Here's how the part is built. I have some questions about the finished solid (model axes, mm). Give positions to 0.01 mm unless a question says otherwise; leave off trailing zeros. Loops run counter-clockwise (first coordinate to the right, second up) from the corner with the lowest first, then second, coordinate; pieces in that order, holes last. Notation, with made-up numbers: (18, -16.75) -> (69, -16.75) arc R12 ccw to (69, 6.25) -> close; hole circle Ø6 at (-11.5, 57). An arc over 180 degrees is marked (long way). Answer in a Markdown table with one row per item. Add a question column.
Item 1: If we section it at D-D (z = 10.5): Write out the boundary of the cut face in (x, y), then the cut area to 3 significant figures.
Item 2: If I drill on line 1 (X direction, y = -1.8, z = 46); line 2 (X direction, y = -0.65, z = 45.5); line 3 (Z direction, x = -18, y = -2.45) (3 decimals), over which ranges is the centre line in solid material (lowest first)?
Item 3: If we section it at C-C (x = 7): Write out the boundary of the cut face in (y, z) (3 decimals).
Item 4: If we section it at B-B (y = -1.2): Write out the boundary of the cut face in (x, z) (3 decimals), then the cut area to 3 significant figures.
Item 5: If we section it at A-A (z = 22.5): Write out the boundary of the cut face in (x, y), then the cut area to 3 significant figures.
Item 6: For P1, Ø1.4, axis at y = -1, z = 11.5, coming from the +X side; P2, Ø1.4, axis at x = -11.5, y = -1, coming from the -Z side; P3, Ø1.4, axis at x = 20, y = -1, coming from the +Z side, each with a flat end and sliding along its axis, tell me the tip position at first contact or that it passes through.
```python
from build123d import *

# Parameters (mm, degrees)
F1_DEPTH = 3.048
F2_SCALE = 0.9


with BuildPart() as f1:
    # F0 (on Front) → F1 (new body)
    with BuildSketch(Plane.XZ):
        Polygon((3.3501721919, 67.3975870013), (0, 67.3975870013), (0, 5.1237931475), (3.3501721919, 5.1237931475), (3.3501721919, 28.9080845579), (24.633621797, 13.3751591098), (27.2410747923, 16.9479306787), (5.6389208675, 32.7134504914), (29.7574140131, 32.7134504914), (29.7574140131, 36.9055655311), (5.6389208675, 36.9055655311), (27.2410747923, 54.3072999545), (24.633621797, 57.5441382825), (3.3501721919, 40.3991378844), align=None)
        Polygon((0, 5.1237931475), (0, 67.3975870013), (-3.3501721919, 67.3975870013), (-3.3501721919, 40.3991378844), (-24.633621797, 57.5441382825), (-27.2410747923, 54.3072999545), (-5.6389208675, 36.9055655311), (-29.7574140131, 36.9055655311), (-29.7574140131, 32.7134504914), (-5.6389208675, 32.7134504914), (-27.2410747923, 16.9479306787), (-24.633621797, 13.3751591098), (-3.3501721919, 28.9080845579), (-3.3501721919, 5.1237931475), align=None)
    extrude(amount=F1_DEPTH)


with BuildPart() as f1_1:
    # F2: moved
    add(f1.part.scale(F2_SCALE))


solid = f1_1.part
```
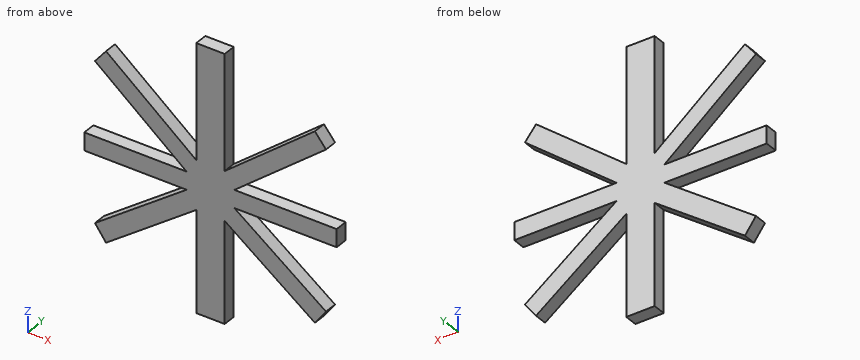
Recorded:
| question | item | result |
|---|---|---|
| 1 | outline | (-3.02, -2.74) -> (3.02, -2.74) -> (3.02, 0) -> (-3.02, 0) -> close |
| 1 | area | 16.5 mm^2 |
| 2 | line 1 | x = -20.95 to -14.98, -3.02 to 3.02, 14.98 to 20.95 |
| 2 | line 2 | x = -20.33 to -14.36, -3.02 to 3.02, 14.36 to 20.33 |
| 2 | line 3 | z = 15.081 to 20.009, 29.442 to 33.215, 43.627 to 48.43 |
| 3 | outline | (-2.743, 23.109) -> (0, 23.109) -> (0, 28.037) -> (-2.743, 28.037) -> close; (-2.743, 29.442) -> (0, 29.442) -> (0, 33.215) -> (-2.743, 33.215) -> close; (-2.743, 34.766) -> (0, 34.766) -> (0, 39.569) -> (-2.743, 39.569) -> close |
| 4 | outline | (-26.782, 29.442) -> (-5.075, 29.442) -> (-24.517, 15.253) -> (-22.17, 12.038) -> (-3.015, 26.017) -> (-3.015, 4.611) -> (3.015, 4.611) -> (3.015, 26.017) -> (22.17, 12.038) -> (24.517, 15.253) -> (5.075, 29.442) -> (26.782, 29.442) -> (26.782, 33.215) -> (5.075, 33.215) -> (24.517, 48.877) -> (22.17, 51.79) -> (3.015, 36.359) -> (3.015, 60.658) -> (-3.015, 60.658) -> (-3.015, 36.359) -> (-22.17, 51.79) -> (-24.517, 48.877) -> (-5.075, 33.215) -> (-26.782, 33.215) -> close |
| 4 | area | 906 mm^2 |
| 5 | outline | (-14.59, -2.74) -> (-7.83, -2.74) -> (-7.83, 0) -> (-14.59, 0) -> close; (-3.02, -2.74) -> (3.02, -2.74) -> (3.02, 0) -> (-3.02, 0) -> close; (7.83, -2.74) -> (14.59, -2.74) -> (14.59, 0) -> (7.83, 0) -> close |
| 5 | area | 53.6 mm^2 |
| 6 | P1 | stops at x = 22.29 |
| 6 | P2 | stops at z = 19.31 |
| 6 | P3 | stops at z = 50.61 |
